Can you work these out from the model? Positions are in its coordinate system, mm. Face numbers are marked on the shaded views. A direction names the side the tool comes from. Round coordinates to 2 decimals unless told otherwise and drop trailing zeros. Loops run counter-clockwise (first coordinate to the right, second up) from the corner with the lowest first, then second, coordinate; pieces in that order, holes last. Notation, with made-up numbers: (74.5, 19) -> (128.5, 19) arc R28 cw to (128.5, 54) -> close; hole circle Ø6 at (-37.75, -38.5). An arc over 180 degrees is marked (long way). Answer as a JSON object with one key per item and string values.
```python
from build123d import *

# Parameters (mm, degrees)
SKETCH2_W           = 8.35
SKETCH2_H           = 8.35
CUT_EXTRUDE1_DEPTH  = 10
SKETCH3_W           = 5.95
SKETCH3_H           = 5.95
BOSS_EXTRUDE1_DEPTH = 10
SKETCH6_W           = 20
SKETCH6_H           = 20
SKETCH6_W_2         = 16
SKETCH6_H_2         = 16
CUT_EXTRUDE2_DEPTH  = 15
CUT_EXTRUDE2_DRAFT  = 6
BOSS_EXTRUDE2_START = 0.3
SKETCH5_R           = 8
BOSS_EXTRUDE2_DEPTH = 0.3


with BuildPart() as part:
    # Sketch1 → Revolve1 (revolve)
    with BuildSketch(Plane.XY):
        Polygon((3.7, 10), (3.7, 0), (4.5, 0), (8, 10), (8, 20.5), (0, 20.5), (0, 10), align=None)
    revolve(axis=Axis((0, 0, 0), (0, 1, 0)))

    # Sketch2 → Cut-Extrude1 (cut)
    with BuildSketch(Plane(origin=(0, 20.5, 0), x_dir=(1, 0, 0), z_dir=(0, 1, 0))):
        Rectangle(SKETCH2_W, SKETCH2_H)
    extrude(amount=-CUT_EXTRUDE1_DEPTH, mode=Mode.SUBTRACT)


with BuildPart() as body_2:
    # Sketch3 → Boss-Extrude1 (new body)
    with BuildSketch(Plane(origin=(0, 10.5, 0), x_dir=(1, 0, 0), z_dir=(0, 1, 0))):
        Rectangle(SKETCH3_W, SKETCH3_H)
    extrude(amount=BOSS_EXTRUDE1_DEPTH)

    # Sketch4 → Cut-Revolve1 (revolve, cut)
    with BuildSketch(Plane.XY, mode=Mode.PRIVATE) as cut_revolve1_sk:
        Polygon((1, 26.5), (7.325, 6.5), (7.325, 26.5), align=None)
    revolve(cut_revolve1_sk.sketch.rotate(Axis((0, 20.5, 0), (0, 1, 0)), 315.000122561), axis=Axis((0, 20.5, 0), (0, 1, 0)), mode=Mode.SUBTRACT)


with BuildPart() as cut_extrude2_tool:
    # Sketch6 → Cut-Extrude2 (with draft: the straight prism first)
    with BuildSketch(Plane(origin=(0, 20.5, 0), x_dir=(1, 0, 0), z_dir=(0, 1, 0))):
        Rectangle(SKETCH6_W, SKETCH6_H)
        Rectangle(SKETCH6_W_2, SKETCH6_H_2, mode=Mode.SUBTRACT)
    extrude(amount=-CUT_EXTRUDE2_DEPTH)
    # Cut-Extrude2: the draft: its side faces are tilted about the plane it starts from
    cut_extrude2_sides = [cut_extrude2_tool.faces().sort_by_distance(p)[0] for p in [
        (-10, 13, 0),
        (0, 13, 10),
        (10, 13, 0),
        (0, 13, -10),
        (0, 13, -8),
        (8, 13, 0),
        (0, 13, 8),
        (-8, 13, 0),
    ]]
    draft(cut_extrude2_sides, Plane(origin=(0, 20.5, 0), x_dir=(1, 0, 0), z_dir=(0, 1, 0)), CUT_EXTRUDE2_DRAFT)


with BuildPart() as part_1:
    add(part.part)

    # Cut-Extrude2: cut by cut_extrude2_tool
    add(cut_extrude2_tool.part, mode=Mode.SUBTRACT)

    # Intersect2: read off the stored shape, not the designer's step
    # Intersect2: union body 2
    add(body_2.part)

    # Sketch5 → Boss-Extrude2 (add)
    with BuildSketch(Plane(origin=(0, 0, 0), x_dir=(1, 0, 0), z_dir=(0, 1, 0)).offset(BOSS_EXTRUDE2_START)):
        with Locations(Location((0, 0, 0), (0, 0, 270))):
            Circle(SKETCH5_R)
    extrude(amount=-BOSS_EXTRUDE2_DEPTH)


solid = part_1.part
```
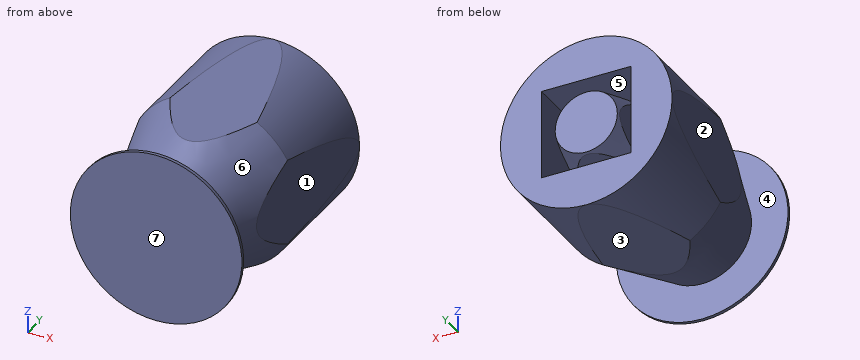
Q1. If I drill on L1, parallel to Z at x = 0, y = 5.5; L2, parallel to Y at x = -1.5, z = 0; L3, parallel to Z at x = -0.25, y = 14.5 (3 decimals), over which ranges is the centre line in solid material (lowest first)? Write a range as [from, to].
Determined:
{"L1": "[-6.42, -3.7], [3.7, 6.42]", "L2": "[0, 0.3], [10, 20.5]", "L3": "[-7.369, -4.175], [-2.975, 2.975], [4.175, 7.369]"}
Q2. We'd pull the mould along Z, two halves only. Please class the marked faces 5, 6 and 7: pulls with the +Z half, pulls with the -Z half, needs draft (parallel to the pull), parting line crosses it, or undercut.
Determined:
{"face 5": "undercut", "face 6": "parting line crosses it", "face 7": "needs draft"}
Q3. I want a section at B-B, the plane y = 6.5. Write out the boundary of the cut face in (x, z) (3 decimals), then the cut area to 3 significant figures.
Determined:
{"outline": "(-6.529, -1.811) arc R6.775 ccw to (-1.811, -6.529) -> (1.811, -6.529) arc R6.775 ccw to (6.529, -1.811) -> (6.529, 1.811) arc R6.775 ccw to (1.811, 6.529) -> (-1.811, 6.529) arc R6.775 ccw to (-6.529, 1.811) -> close; hole circle Ø7.4 at (0, 0)", "area": "98.8 mm²"}
Q4. I want a section at A-A, the plane y = 15. Write out the boundary of the cut face in (x, z) (3 decimals).
Determined:
{"outline": "(-7.422, -2.986) arc R8 ccw to (-2.986, -7.422) -> (2.986, -7.422) arc R8 ccw to (7.422, -2.986) -> (7.422, 2.986) arc R8 ccw to (2.986, 7.422) -> (-2.986, 7.422) arc R8 ccw to (-7.422, 2.986) -> close; (-2.975, -2.975) -> (2.975, -2.975) -> (2.975, 2.975) -> (-2.975, 2.975) -> close; hole (-4.175, -4.175) -> (4.175, -4.175) -> (4.175, 4.175) -> (-4.175, 4.175) -> close"}
Q5. I'm going to push flat-ended pins straight in: pin 1 (5 mm diameter, centred on x = -3.5, z = -3.5, fed in from +Y); pin 2 (5 mm diameter, centred on y = 13.5, z = -1.5, fed in from +X); pin 3 (4 mm diameter, centred on x = -4, y = 9.5, fed in from -Z); pin 4 (9 mm diameter, centred on x = -1, y = 16, fed in from -Z). Where does each tip first touch, or does it pass through?
Determined:
{"pin 1": "y = 20.5", "pin 2": "x = 7.53", "pin 3": "z = -7.05", "pin 4": "z = -7.99"}
Q6. I want a section at C-C, the plane y = 17.25. Write out the boundary of the cut face in (x, z) (3 decimals).
Determined:
{"outline": "(-7.658, -2.313) arc R8 ccw to (-2.313, -7.658) -> (2.313, -7.658) arc R8 ccw to (7.658, -2.313) -> (7.658, 2.313) arc R8 ccw to (2.313, 7.658) -> (-2.313, 7.658) arc R8 ccw to (-7.658, 2.313) -> close; (-2.975, -2.561) arc R3.925 ccw to (-2.561, -2.975) -> (2.561, -2.975) arc R3.925 ccw to (2.975, -2.561) -> (2.975, 2.561) arc R3.925 ccw to (2.561, 2.975) -> (-2.561, 2.975) arc R3.925 ccw to (-2.975, 2.561) -> close; hole (-4.175, -4.175) -> (4.175, -4.175) -> (4.175, 4.175) -> (-4.175, 4.175) -> close"}
Q7. On a 3-axis mill with a long thin cutter (end or side, diameter ignored), from which of +Z, -Z, +X, -X, +Y, -Y can I reach the whole of each face in a straight line? I mean the marked faces 1, 2, 3 and 4. Say none if no direction works.
Determined:
{"face 1": "+Z, -Z, +X", "face 2": "+Z, -Z, -X", "face 3": "-Z, +X, -X", "face 4": "none"}
